Design review of the part built by this model. Coordinates are the model's own, in mm. A direction names the side the tool comes from. Coordinates: 2 decimals unless noted, no trailing zeros. One line per question, with ' | ' between items.
from build123d import *

# Parameters (mm, degrees)
SKETCH019_R             = 106.07
PAD010_DEPTH            = 8.5
SKETCH020_R             = 100
POCKET001_DEPTH         = 7
CHAMFER008_SIZE         = 3
CHAMFER015_SIZE         = 3
SKETCH028_R             = 80
SKETCH028_R_2           = 79
PAD012_DEPTH            = 8
SKETCH029_R             = 1
POCKET006_DEPTH         = 87.5
SKETCH030_R             = 1
POCKET007_DEPTH         = 87.5
CHAMFER016_SIZE         = 1
CHAMFER017_SIZE         = 0.8
CHAMFER018_SIZE         = 0.5
BODY008_PLACEMENT_ANGLE = 180


with BuildPart() as part:
    # Sketch019 → Pad010 (new body)
    with BuildSketch(Plane.XY):
        Circle(SKETCH019_R)
    extrude(amount=PAD010_DEPTH)

    # Sketch020 → Pocket001 (cut)
    with BuildSketch(Plane.XY):
        Circle(SKETCH020_R)
    extrude(amount=POCKET001_DEPTH, mode=Mode.SUBTRACT)

    # Chamfer008
    chamfer008_edges = [part.edges().sort_by_distance(p)[0] for p in [
        (-106.07, 0, 8.5),
    ]]
    chamfer(chamfer008_edges, length=CHAMFER008_SIZE)

    # Chamfer015
    chamfer015_edges = [part.edges().sort_by_distance(p)[0] for p in [
        (-106.07, 0, 0),
    ]]
    chamfer(chamfer015_edges, length=CHAMFER015_SIZE)

    # Sketch028 → Pad012 (join)
    with BuildSketch(Plane.XY):
        Circle(SKETCH028_R)
        Circle(SKETCH028_R_2, mode=Mode.SUBTRACT)
    extrude(amount=PAD012_DEPTH)

    # Sketch029 → Pocket006 (cut, symmetric)
    with BuildSketch(Plane.XZ):
        with Locations((0, 4)):
            Circle(SKETCH029_R)
    extrude(amount=POCKET006_DEPTH, both=True, mode=Mode.SUBTRACT)

    # Sketch030 → Pocket007 (cut, symmetric)
    with BuildSketch(Plane.YZ):
        with Locations((0, 4)):
            Circle(SKETCH030_R)
    extrude(amount=POCKET007_DEPTH, both=True, mode=Mode.SUBTRACT)

    # Chamfer016
    chamfer016_edges = [part.edges().sort_by_distance(p)[0] for p in [
        (-79, 0, 7),
    ]]
    chamfer(chamfer016_edges, length=CHAMFER016_SIZE)

    # Chamfer017
    chamfer017_edges = [part.edges().sort_by_distance(p)[0] for p in [
        (-100, 0, 0),
    ]]
    chamfer(chamfer017_edges, length=CHAMFER017_SIZE)

    # Chamfer018
    chamfer018_edges = [part.edges().sort_by_distance(p)[0] for p in [
        (-80, 0, 0),
    ]]
    chamfer(chamfer018_edges, length=CHAMFER018_SIZE)


with BuildPart() as part_1:
    # Body008 placement: moved
    add(part.part.moved(Location((0, 0, -171))).rotate(Axis((0, 0, -171), (0, 1, 0)), BODY008_PLACEMENT_ANGLE))


solid = part_1.part
Q1. Draft analysis for pull direction X (two halves, no side actions). For faces 3 (the flat face through (1, 1, -179.5)), 4 (the cylindrical face through (-95.38, 30.04, -174.86)), 5 (the cylindrical face through (22.99, -103.55, -175.23)), state which applies: +X half, -X half, draft (parallel to the pull), parting line (faces both ways), or undercut.
Returned:
face 3: draft | face 4: undercut | face 5: parting line
Q2. For pin 1 (5 mm diameter, centred on y = -77.5, z = -174, fed in from +X); pin 2 (8 mm diameter, centred on x = 60.5, y = 68.5, fed in from +Z), all flat-tipped, find the tip position at first contact; note any pin that passes through.
Returned:
pin 1: stops at x = 75.01 | pin 2: stops at z = -178
Q3. Tool access review of faces 1 (the flat face through (-22, -99, -171)), 2 (the flat face through (1, 1, -178)): name each direction out of +Z, -Z, +X, -X, +Y, -Y from which nothing blocks a thin tool from reaching the whole face with its end or side.
Returned:
face 1: +Z, +X, -X, +Y, -Y | face 2: +Z
Q4. To check wall thickness, follow line 1 along X through (y, z) = (18, -172.75); line 2 along Y through (x, z) = (0, -175.75); line 3 along Y through (x, z) = (-12.5, -177.5). State the ranges of each line that lie inside material, in increasing order.
Returned:
line 1: x = -103.26 to -98.37, -77.95 to -76.92, 76.92 to 77.95, 98.37 to 103.26 | line 2: y = -106.07 to -100, 100 to 106.07 | line 3: y = -104.32 to -99.22, -79.02 to -77.5, 77.5 to 79.02, 99.22 to 104.32
